from build123d import *

# Parameters (mm, degrees)
F0_W     = 76.2
F0_H     = 76.2
F1_DEPTH = 76.2
F2_W     = 25.4
F2_H     = 25.4
F3_DEPTH = 12.7
F4_R     = 12.7
F5_DEPTH = 12.7
F7_D     = 25.4
F9_DEPTH = 12.7


with BuildPart() as f1:
    # F0 (on Front) → F1 (new body)
    with BuildSketch(Plane.XZ):
        with Locations((-3.697144, -5.31157)):
            Rectangle(F0_W, F0_H)
    extrude(amount=-F1_DEPTH)

    # F2 (on face) → F3 (join)
    with BuildSketch(Plane.XZ):
        with Locations((-3.697144, 1.963377)):
            Rectangle(F2_W, F2_H)
    extrude(amount=F3_DEPTH)

    # F4 (on face) → F5 (join)
    with BuildSketch(Plane.YZ.offset(34.402856)):
        with Locations((38.1, -5.31157)):
            Circle(F4_R)
    extrude(amount=F5_DEPTH)

    # F7 (through all)
    with Locations(Plane.XY.offset(32.78843)):
        with Locations((0, 38.1)):
            Hole(F7_D / 2)

    # F8 (on face) → F9 (join)
    with BuildSketch(Plane(origin=(-41.797144, 0, 0), x_dir=(0, -1, 0), z_dir=(-1, 0, 0))):
        Polygon((-59.184786, -0.260271), (-31.93216, -26.097179), (-23.183054, 10.422741), align=None)
    extrude(amount=F9_DEPTH)


solid = f1.part
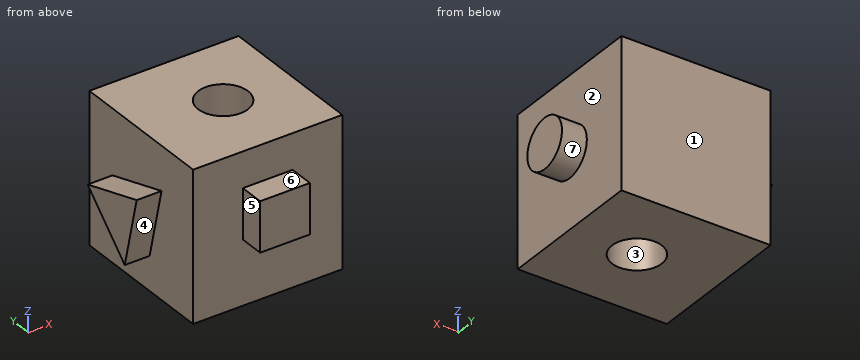
Check sheet for the modelled part. Datum: model origin and axes. Units: mm. Face numbers are marked on the shaded views. A direction names the side the tool comes from. Round coordinates to 2 decimals unless told otherwise and drop trailing zeros. Loops run counter-clockwise (first coordinate to the right, second up) from the corner with the lowest first, then second, coordinate; pieces in that order, holes last. Notation, with made-up numbers: (3, -19) -> (10, -19) arc R18 cw to (10, -13) -> close; hole circle Ø3 at (36, -21.5). An arc over 180 degrees is marked (long way). Put each result on its own line as item: value. Start each with the question number.
1. Section check A-A (x = 0). Enter the section's corners in (y, z).
2. Draft check along X on the marked faces 1, 2 and 3. Enter one of: +X half, -X half, draft (parallel to the pull), parting line (faces both ways), or undercut.
3. Gauge pin test, flat ends, axial feed: pin 1 (2 mm diameter, centred on y = 28.5, z = -31.5, fed in from -X); pin 2 (12 mm diameter, centred on x = -20, z = -21.5, fed in from -Y); pin 3 (10 mm diameter, centred on x = 2, y = -8.5, fed in from +Z). Record the tip position at first contact, or that the pin passes through.
4. Access from +Z, -Z, +X, -X, +Y, -Y to the whole of each face (thin tool, end or side, straight path). Record for the marked faces 4, 5, 6 and 7.
5. Section check D-D (y = 55). Enter the section's corners in (x, z).
6. Scan lines: probe 1 along X at (y, z) = (38, -16); probe 2 along X at (y, z) = (38, -23); probe 3 along Y at (x, z) = (0, 9). Record each from-to range of solid material in increasing order.
7. Section check C-C (z = 1). Enter the section's corners in (x, y), plus the area to 3 significant figures.
8. Section check B-B (y = 38.1). Enter the section's corners in (x, z), plus the area to 3 significant figures.
Findings:
1. outline: (-12.7, -10.74) -> (0, -10.74) -> (0, -43.41) -> (25.4, -43.41) -> (25.4, 32.79) -> (0, 32.79) -> (0, 14.66) -> (-12.7, 14.66) -> close; (50.8, -43.41) -> (76.2, -43.41) -> (76.2, 32.79) -> (50.8, 32.79) -> close
2. face 1: draft
2. face 2: +X half
2. face 3: undercut
3. pin 1: stops at x = -41.8
3. pin 2: stops at y = 0
3. pin 3: stops at z = 14.66
4. face 4: -Z, -X, -Y
4. face 5: +Z, -Z, -X, -Y
4. face 6: +Z, +X, -X, -Y
4. face 7: +X
5. outline: (-54.5, -4.23) -> (-41.8, -4.23) -> (-41.8, -43.41) -> (34.4, -43.41) -> (34.4, 32.79) -> (-41.8, 32.79) -> (-41.8, 0.98) -> (-54.5, 0.98) -> close
6. probe 1: x = -54.5 to -12.7, 12.7 to 47.1
6. probe 2: x = -41.8 to -12.7, 12.7 to 34.4
6. probe 3: y = -12.7 to 25.4, 50.8 to 76.2
7. outline: (-54.5, 25.44) -> (-41.8, 25.44) -> (-41.8, 0) -> (-16.4, 0) -> (-16.4, -12.7) -> (9, -12.7) -> (9, 0) -> (34.4, 0) -> (34.4, 27.08) -> (47.1, 27.08) -> (47.1, 49.12) -> (34.4, 49.12) -> (34.4, 76.2) -> (-41.8, 76.2) -> (-41.8, 54.94) -> (-54.5, 54.94) -> close; hole circle Ø25.4 at (0, 38.1)
7. area: 6,280 mm^2
8. outline: (-54.5, -20.25) -> (-41.8, -20.25) -> (-41.8, -43.41) -> (-12.7, -43.41) -> (-12.7, 32.79) -> (-41.8, 32.79) -> (-41.8, 6) -> (-54.5, 6) -> close; (12.7, -43.41) -> (34.4, -43.41) -> (34.4, -18.01) -> (47.1, -18.01) -> (47.1, 7.39) -> (34.4, 7.39) -> (34.4, 32.79) -> (12.7, 32.79) -> close
8. area: 4,530 mm^2
